Here's the drawing with two shaded views (mm, measured from the low corner). I have some questions. A direction names the side the tool comes from. Give positions to 0.01 mm unless a question says otherwise; leave off trailing zeros. Loops run counter-clockwise (first coordinate to the right, second up) from the corner with the lowest first, then second, coordinate; pieces in that order, holes last. Notation, with made-up numbers: M 15,-18 L 52,-18 A13 cw 52,-10 Z; hole C 39.25,40.5 d4. An arc over 180 degrees is marked long. Answer in a Markdown table with one row per item. Add a question column.
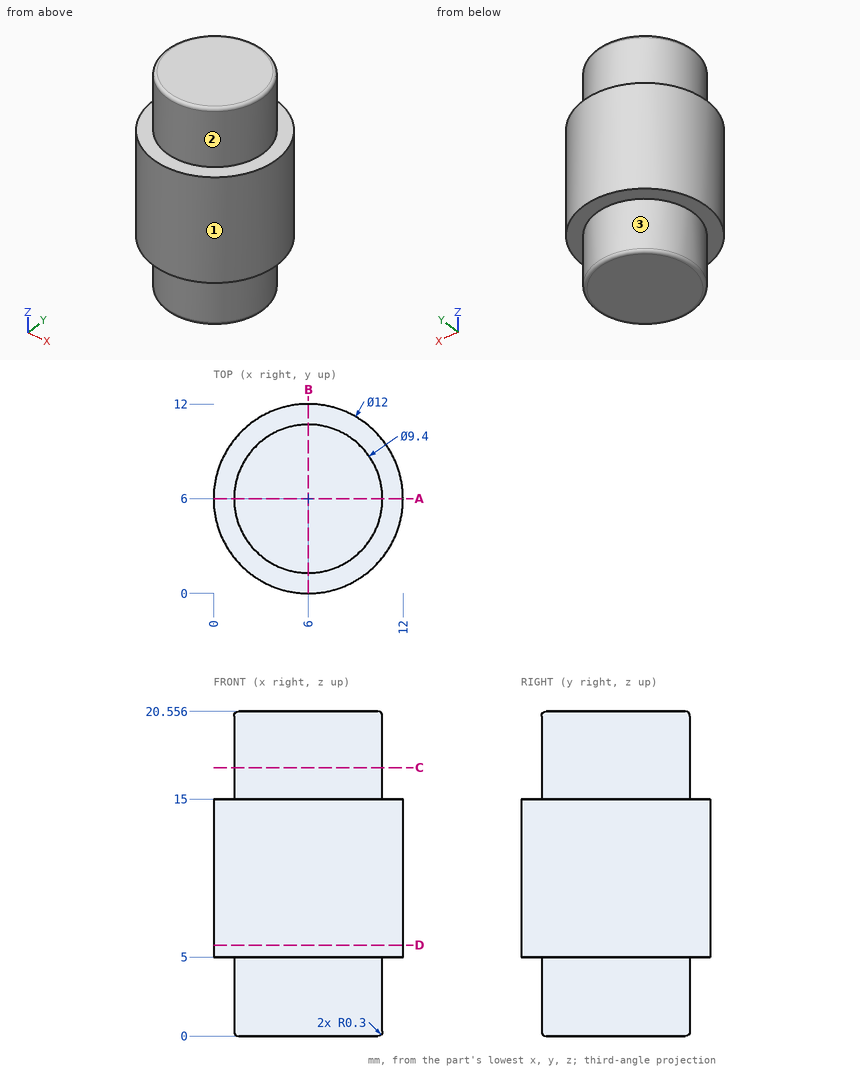
Item 1: I need wall thicknesses on L1, parallel to Z at x = 0.75, y = 6.5; L2, parallel to Y at x = 6, z = 2.5; L3, parallel to X at y = 4.75, z = 7. Which ranges of each line are inside material? Lowest first, please.
Item 2: Suppose I cut it at A-A (y = 6). List the corners of the cut face in (x, z) for me.
Item 3: Suppose I cut it at D-D (z = 5.75). List the corners of the cut face in (x, y) for me.
Item 4: Suppose I cut it at C-C (z = 17). List the corners of the cut face in (x, y) for me.
Item 5: For the marked faces 1, 2 and 3, which set-ups out of +Z, -Z, +X, -X, +Y, -Y let a thin tool reach every point of the face, with its end or its side?
Values found:
| question | item | result |
|---|---|---|
| 1 | L1 | 5 to 15 |
| 1 | L2 | 1.3 to 10.7 |
| 1 | L3 | 0.13 to 11.87 |
| 2 | outline | M 0,5 L 1.3,5 L 1.3,0.3 A0.3 ccw 1.6,0 L 10.4,0 A0.3 ccw 10.7,0.3 L 10.7,5 L 12,5 L 12,15 L 10.7,15 L 10.7,20.26 A0.3 ccw 10.4,20.56 L 1.6,20.56 A0.3 ccw 1.3,20.26 L 1.3,15 L 0,15 Z |
| 3 | outline | C 6,6 d12 |
| 4 | outline | C 6,6 d9.4 |
| 5 | face 1 | +Z, -Z |
| 5 | face 2 | +Z |
| 5 | face 3 | -Z |
